from build123d import *

# Parameters (mm, degrees)
BOSS_EXTRUDE1_DEPTH = 30
BOSS_EXTRUDE2_DEPTH = 30
CUT_EXTRUDE1_DEPTH  = 64
SKETCH4_R           = 25
CUT_EXTRUDE2_DEPTH  = 93
SKETCH6_W           = 50
SKETCH6_H           = 99.213444665
BOSS_EXTRUDE3_DEPTH = 100


with BuildPart() as part:
    # Sketch1 → Boss-Extrude1 (new body)
    with BuildSketch(Plane.XY):
        with BuildLine():
            Line((-100, 25), (-143.301270189, 25))
            ThreePointArc((-143.301270189, 25), (-125, 43.301270189), (-100, 50))
            Line((-100, 50), (0, 50))
            Line((0, 50), (0, 15))
            Line((0, 15), (100, 15))
            Line((100, 15), (100, -15))
            Line((100, -15), (0, -15))
            Line((0, -15), (0, -50))
            Line((0, -50), (-100, -50))
            ThreePointArc((-100, -50), (-125, -43.301270189), (-143.301270189, -25))
            Line((-143.301270189, -25), (-100, -25))
            ThreePointArc((-100, -25), (-75, 0), (-100, 25))
        make_face()
    extrude(amount=-BOSS_EXTRUDE1_DEPTH)

    # Sketch2 → Boss-Extrude2 (add)
    with BuildSketch(Plane(origin=(0, 15, 0), x_dir=(1, 0, 0), z_dir=(0, 1, 0))):
        with BuildLine():
            Line((49.998729811, 65), (-0.001270189, 65))
            Line((-0.001270189, 65), (-0.001270189, -35))
            Line((-0.001270189, -35), (49.998729811, -35))
            ThreePointArc((49.998729811, -35), (99.998729811, 15), (49.998729811, 65))
        make_face()
    extrude(amount=-BOSS_EXTRUDE2_DEPTH)

    # Sketch3 → Cut-Extrude1 (cut)
    with BuildSketch(Plane(origin=(0, 15, 0), x_dir=(1, 0, 0), z_dir=(0, 1, 0))):
        with BuildLine():
            Line((97.695689882, 30), (100, 30))
            Line((100, 30), (100, 0))
            Line((100, 0), (97.695689882, 0))
            ThreePointArc((97.695689882, 0), (99.998729811, 15), (97.695689882, 30))
        make_face()
    extrude(amount=-CUT_EXTRUDE1_DEPTH, mode=Mode.SUBTRACT)

    # Sketch4 → Cut-Extrude2 (cut)
    with BuildSketch(Plane(origin=(0, 15, 0), x_dir=(1, 0, 0), z_dir=(0, 1, 0))):
        with Locations(Location((49.998729811, 15, 0), (0, 0, 270))):
            Circle(SKETCH4_R)
    extrude(amount=-CUT_EXTRUDE2_DEPTH, mode=Mode.SUBTRACT)

    # Sketch6 → Boss-Extrude3 (add)
    with BuildSketch(Plane(origin=(0, 50, 0), x_dir=(1, 0, 0), z_dir=(0, 1, 0))):
        with Locations((-25.001270189, 15.393277667)):
            Rectangle(SKETCH6_W, SKETCH6_H)
    extrude(amount=-BOSS_EXTRUDE3_DEPTH)


solid = part.part
Geometry check sheet. Reference: the model listing, model coordinates, mm. A direction names the side the tool comes from. Give positions to 0.01 mm unless a question says otherwise; leave off trailing zeros. Loops run counter-clockwise (first coordinate to the right, second up) from the corner with the lowest first, then second, coordinate; pieces in that order, holes last. Notation, with made-up numbers: M 64,6 L 95,6 A18 ccw 95,12 Z; hole C 73.5,33.25 d9. An arc over 180 degrees is marked long. Write each question's results on one line, items separated by ' | '.
1) Section check C-C, the plane x = 63. Record the boundary of the cut face in (y, z), plus the area to 3 significant figures.
Answers follow:
outline: M -15,-63.28 L 15,-63.28 L 15,-36.35 L -15,-36.35 Z; M -15,6.35 L 15,6.35 L 15,33.28 L -15,33.28 Z | area: 1,620 mm2
2) Tool access check on faces 5 (the face through (-75, -10, 0)), 6 (the face through (0, 33, -15)), 7 (the face through (-75, -10, -30)), 8 (the face through (-0.001, -32, -47)), 9 (the face through (-122, -25, -15)). Record the directions out of +Z, -Z, +X, -X, +Y, -Y that give a thin tool (end or side, any length) a straight path to the whole face; none if there is none.
Answers follow:
face 5: +Z, -X, +Y, -Y | face 6: +Z, -Z, +X, +Y | face 7: -Z, -X, +Y, -Y | face 8: +Z, -Z, +X, -Y | face 9: +Z, -Z, -X
3) Release check for a two-part mould opening along Y. For faces 1 (the face through (-121, 25, -15)), 2 (the face through (-75.006, -0.55, -14.79)), 3 (the face through (27, 15, -27)), 4 (the face through (-50.001, 1, -47)) record: +Y half, -Y half, draft (parallel to the pull), parting line (faces both ways), or undercut.
Answers follow:
face 1: undercut | face 2: undercut | face 3: +Y half | face 4: draft
4) Gauge pin test, flat ends, axial feed: pin 1 (9 mm diameter, centred on y = 30.5, z = -7.5, fed in from +X); pin 2 (12 mm diameter, centred on x = 0.5, z = 14.5, fed in from -Y); pin 3 (1.5 mm diameter, centred on x = -105.5, y = 38.5, fed in from +Z); pin 4 (15 mm diameter, centred on x = -130, z = -18.5, fed in from +Y). Record the tip position at first contact, or that the pin passes through.
Answers follow:
pin 1: x = 0 | pin 2: y = -50 | pin 3: z = 0 | pin 4: y = 44.65
5) Section check B-B, the plane y = 12. Record the boundary of the cut face in (x, z).
Answers follow:
outline: M -78.07,-30 L -50,-30 L -50,-65 L 50,-65 A50 ccw 50,35 L 0,35 L 0,34.21 L -50,34.21 L -50,0 L -78.07,0 Z; hole C 50,-15 d50
6) Thickness scan on line 1 (X direction, y = -41, z = 11.5); line 2 (Z direction, x = -116, y = 34.5); line 3 (Z direction, x = -12, y = 4.5). Record the ranges inside material, lowest first.
Answers follow:
line 1: -50 to 0 | line 2: -30 to 0 | line 3: -65 to 34.21
7) Section check A-A, the plane z = -15. Record the boundary of the cut face in (x, y), plus the area to 3 significant figures.
Answers follow:
outline: M -143.3,-25 A50 ccw -100,-50 L 0,-50 L 0,-15 L 25,-15 L 25,15 L 0,15 L 0,50 L -100,50 A50 ccw -143.3,25 L -100,25 A25 cw -100,-25 Z; M 75,-15 L 100,-15 L 100,15 L 75,15 Z | area: 12,100 mm2
